from build123d import *

# Parameters (mm, degrees)
SKETCH1_R           = 10
BOSS_EXTRUDE1_DEPTH = 17
SKETCH2_W           = 16
SKETCH2_H           = 120
BOSS_EXTRUDE2_DEPTH = 100
FILLET1_R           = 8
SKETCH3_R           = 8.5
BOSS_EXTRUDE3_DEPTH = 25
RIB2_REACH          = 167.497
SKETCH6_WALL_W      = 455.059513806
SKETCH6_WALL_H      = 15
FILLET2_R           = 4
FILLET3_R           = 8


with BuildPart() as part:
    # Sketch1 → Boss-Extrude1 (new body)
    with BuildSketch(Plane(origin=(0, 0, 0), x_dir=(1, 0, 0), z_dir=(0, 1, 0))):
        with BuildLine():
            Line((-30.5, 60), (30.5, 60))
            Line((30.5, 60), (30.5, -60))
            Line((30.5, -60), (-30.5, -60))
            ThreePointArc((-30.5, -60), (-48.17766953, -52.67766953), (-55.5, -35))
            Line((-55.5, -35), (-55.5, 35))
            ThreePointArc((-55.5, 35), (-48.17766953, 52.67766953), (-30.5, 60))
        make_face()
        with Locations(Location((-30.5, 35, 0), (0, 0, 270))):
            Circle(SKETCH1_R, mode=Mode.SUBTRACT)
        with Locations(Location((-30.5, -35, 0), (0, 0, 270))):
            Circle(SKETCH1_R, mode=Mode.SUBTRACT)
    extrude(amount=BOSS_EXTRUDE1_DEPTH)

    # Sketch2 → Boss-Extrude2 (add)
    with BuildSketch(Plane(origin=(0, 17, 0), x_dir=(1, 0, 0), z_dir=(0, 1, 0))):
        with Locations((22.5, 0)):
            Rectangle(SKETCH2_W, SKETCH2_H)
    extrude(amount=BOSS_EXTRUDE2_DEPTH)

    # Fillet1
    fillet1_edges = [part.edges().sort_by_distance(p)[0] for p in [
        (14.5, 17, 0),
    ]]
    fillet(fillet1_edges, radius=FILLET1_R)

    # Sketch3 → Boss-Extrude3 (add)
    with BuildSketch(Plane(origin=(0, 117, 0), x_dir=(1, 0, 0), z_dir=(0, 1, 0))):
        with BuildLine():
            Line((30.5, 60), (82.727979275, 30.466321244))
            ThreePointArc((82.727979275, 30.466321244), (100.5, 0), (82.727979275, -30.466321244))
            Line((82.727979275, -30.466321244), (30.5, -60))
            Line((30.5, -60), (30.5, 60))
        make_face()
        with Locations(Location((65.5, 0, 0), (0, 0, 270))):
            Circle(SKETCH3_R, mode=Mode.SUBTRACT)
    extrude(amount=-BOSS_EXTRUDE3_DEPTH)

    # Sketch6 wall → Rib2 (add, up to next)
    with BuildSketch(Plane(origin=(-20.5, 67, 0), x_dir=(-0.573462344363, -0.819231920519, 0), z_dir=(0.819231920519, -0.573462344363, 0)), mode=Mode.PRIVATE) as rib2_sk1:
        Rectangle(SKETCH6_WALL_W, SKETCH6_WALL_H)
    rib2_tool1 = extrude(rib2_sk1.sketch, amount=RIB2_REACH, mode=Mode.PRIVATE) - part.part
    add(rib2_tool1.solids().sort_by_distance((-20.5, 67, 0))[0])

    # Fillet2
    fillet2_edges = [part.edges().sort_by_distance(p)[0] for p in [
        (12.156854249, 19.343145751, -7.5),
        (-24.5, 17, -7.5),
        (14.5, 71, -7.5),
        (12.156854249, 19.343145751, 7.5),
        (-24.5, 17, 7.5),
        (14.5, 71, 7.5),
    ]]
    fillet(fillet2_edges, radius=FILLET2_R)

    # Fillet3
    fillet3_edges = [part.edges().sort_by_distance(p)[0] for p in [
        (30.5, 92, 0),
    ]]
    fillet(fillet3_edges, radius=FILLET3_R)


solid = part.part
Here's how the part is built. I have some questions about the finished solid (model axes, mm). A direction names the side the tool comes from. Give positions to 0.01 mm unless a question says otherwise; leave off trailing zeros. Loops run counter-clockwise (first coordinate to the right, second up) from the corner with the lowest first, then second, coordinate; pieces in that order, holes last. Notation, with made-up numbers: (35, 49) -> (56, 49) arc R4 cw to (56, 55) -> close; hole circle Ø3 at (-11, 83). An arc over 180 degrees is marked (long way). Answer as a JSON object with one key per item and string values. Group by question number.
Item 1: Imagine slicing it at D-D on x = -43. Write out the boundary of the cut face in (y, z), then the cut area to 3 significant figures.
Item 2: I need wall thicknesses on L1, parallel to Z at x = -30, y = 8; L2, parallel to X at y = 4, z = 35; L3, parallel to X at y = 44.5, z = -26.5. Which ranges of each line are inside material? Lowest first, please.
Item 3: Imagine slicing it at C-C on x = 65.5. Write out the boundary of the cut face in (y, z), then the cut area to 3 significant figures.
Item 4: Thinking about a two-plate mould opening in X: for faces 1 (the cylindrical face through (32.906, 89.719, -0.84)), 2 (the cylindrical face through (73.928, 104.675, -1.107)), 3 (the flat face through (16, 50, -60)), which applies, pulls with the +X half, pulls with the -X half, needs draft (parallel to the pull), parting line crosses it, or undercut?
Item 5: On a 3-axis mill with a long thin cutter (end or side, diameter ignored), from which of +Z, -Z, +X, -X, +Y, -Y can I reach the whole of each face in a straight line? I mean faces 4 (the flat face through (-17, 49, 7.5)), 5 (the flat face through (56.25, 104.4, -45.44)), 6 (the flat face through (-17, 17, -36)). Say none if no direction works.
Item 6: Imagine slicing it at B-B on y = 36. Write out the boundary of the cut face in (x, z), then the cut area to 3 significant figures.
Item 7: Will these pins go through, and if not, where does the flat tip stop? pin 1 (23 mm diameter, centred on x = -30.5, z = -35, fed in from +Y); pin 2 (19 mm diameter, centred on x = -8, y = 86.5, fed in from -Z); pin 3 (5 mm diameter, centred on y = 52.5, z = 1, fed in from +X).
Item 8: Imagine slicing it at A-A on z = 0. Write out the boundary of the cut face in (x, y), then the cut area to 3 significant figures.
Answer list:
{
 "1": {"outline": "(0, -56.65) -> (17, -56.65) -> (17, -11.5) arc R4 cw to (21, -7.5) -> (34.86, -7.5) -> (34.86, 7.5) -> (21, 7.5) arc R4 cw to (17, 11.5) -> (17, 56.65) -> (0, 56.65) -> close", "area": "2,200 mm2"},
 "2": {"L1": "z = -60 to -44.99, -25.01 to 25.01, 44.99 to 60", "L2": "x = -55.5 to -40.5, -20.5 to 30.5", "L3": "x = 14.5 to 30.5"},
 "3": {"outline": "(92, -40.21) -> (117, -40.21) -> (117, -8.5) -> (92, -8.5) -> close; (92, 8.5) -> (117, 8.5) -> (117, 40.21) -> (92, 40.21) -> close", "area": "1,590 mm2"},
 "4": {"face 1": "pulls with the +X half", "face 2": "undercut", "face 3": "needs draft"},
 "5": {"face 4": "+Z, -X, +Y", "face 5": "-Z, +X, +Y, -Y", "face 6": "-Z, -X, +Y"},
 "6": {"outline": "(-42.2, -7.5) -> (10.5, -7.5) arc R4 cw to (14.5, -11.5) -> (14.5, -60) -> (30.5, -60) -> (30.5, 60) -> (14.5, 60) -> (14.5, 11.5) arc R4 cw to (10.5, 7.5) -> (-42.2, 7.5) -> close", "area": "2,780 mm2"},
 "7": {"pin 1": "stops at y = 17", "pin 2": "stops at z = -7.5", "pin 3": "stops at x = 30.5"},
 "8": {"outline": "(-55.5, 0) -> (30.5, 0) -> (30.5, 84) arc R8 cw to (38.5, 92) -> (57, 92) -> (57, 117) -> (14.5, 117) -> (-55.5, 17) -> close; (74, 92) -> (100.5, 92) -> (100.5, 117) -> (74, 117) -> close", "area": "7,900 mm2"}
}
